Geometry check sheet. Reference: drawing and pictorial views, mm from the part's lowest x, y, z. A direction names the side the tool comes from. Give positions to 0.01 mm unless a question says otherwise; leave off trailing zeros. Loops run counter-clockwise (first coordinate to the right, second up) from the corner with the lowest first, then second, coordinate; pieces in that order, holes last. Notation, with made-up numbers: (-38, 42.25) - (21, 42.25) arc R26 ccw to (21, 61.25) - close; hole circle Ø9 at (26.25, -11). An arc over 180 degrees is marked (long way). Answer in a Markdown table with one row per item. Add a question column.
(1) Sectioned sample at B-B on x = 14.5. Enter the section's corners in (y, z).
(2) Sectioned sample at A-A on y = 60.5. Enter the section's corners in (x, z).
(3) Sectioned sample at C-C on z = 24.5. Enter the section's corners in (x, y), then the cut area to 3 significant figures.
(4) Set-up check for the marked faces 4 and 5: record each of +Z, -Z, +X, -X, +Y, -Y from which the full face is reachable in a straight line by a thin tool's end or side.
(5) Draft check along X on the marked faces 1, 2 and 3. Enter one of: released by +X, released by -X, zero draft, split by the parting line, or undercut.
(6) Sectioned sample at D-D on x = 35. Enter the section's corners in (y, z).
(7) Thickness scan on L1, parallel to X at y = 32, z = 21.5; L2, parallel to Y at x = 35, z = 15; L3, parallel to Y at x = 18, z = 35. Record the ranges inside material, lowest first.
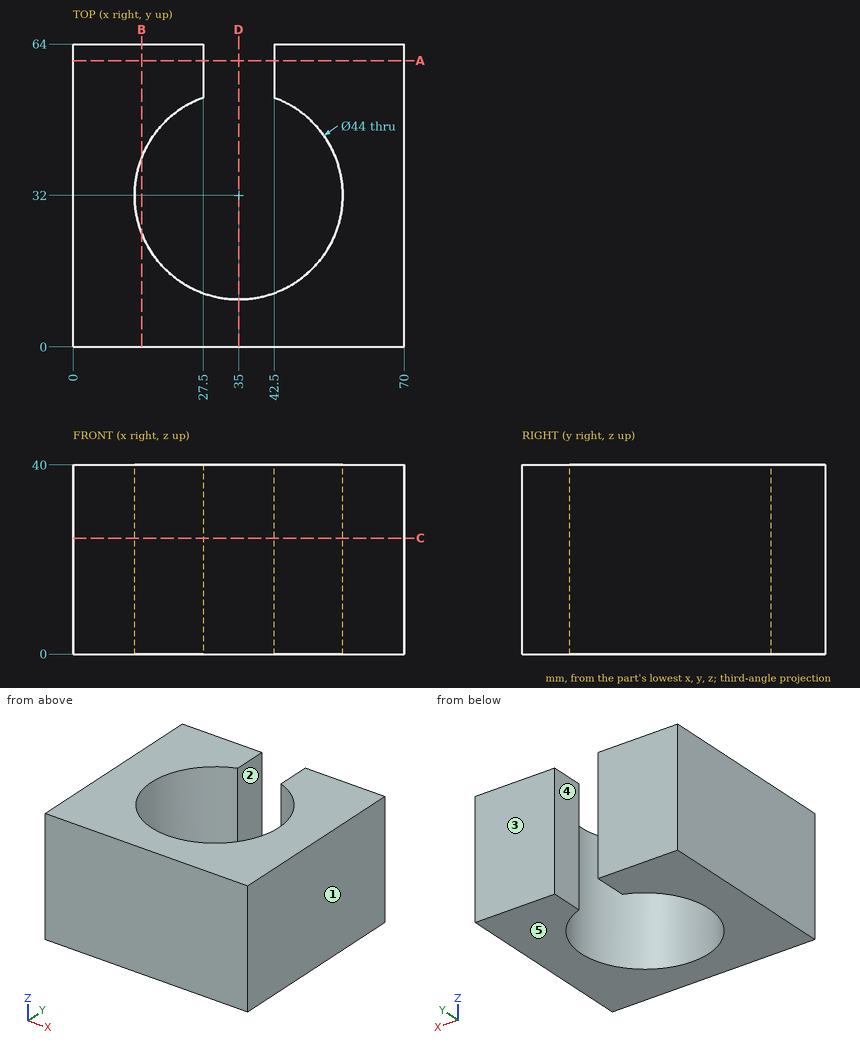
Reply:
| question | item | result |
|---|---|---|
| 1 | outline | (0, 0) - (24.02, 0) - (24.02, 40) - (0, 40) - close; (39.98, 0) - (64, 0) - (64, 40) - (39.98, 40) - close |
| 2 | outline | (0, 0) - (27.5, 0) - (27.5, 40) - (0, 40) - close; (42.5, 0) - (70, 0) - (70, 40) - (42.5, 40) - close |
| 3 | outline | (0, 0) - (70, 0) - (70, 64) - (42.5, 64) - (42.5, 52.68) arc R22 cw (long way) to (27.5, 52.68) - (27.5, 64) - (0, 64) - close |
| 3 | area | 2,800 mm^2 |
| 4 | face 4 | +Z, -Z, +Y |
| 4 | face 5 | -Z, +X, -X, +Y, -Y |
| 5 | face 1 | released by +X |
| 5 | face 2 | undercut |
| 5 | face 3 | zero draft |
| 6 | outline | (0, 0) - (10, 0) - (10, 40) - (0, 40) - close |
| 7 | L1 | 0 to 13, 57 to 70 |
| 7 | L2 | 0 to 10 |
| 7 | L3 | 0 to 18.04, 45.96 to 64 |
